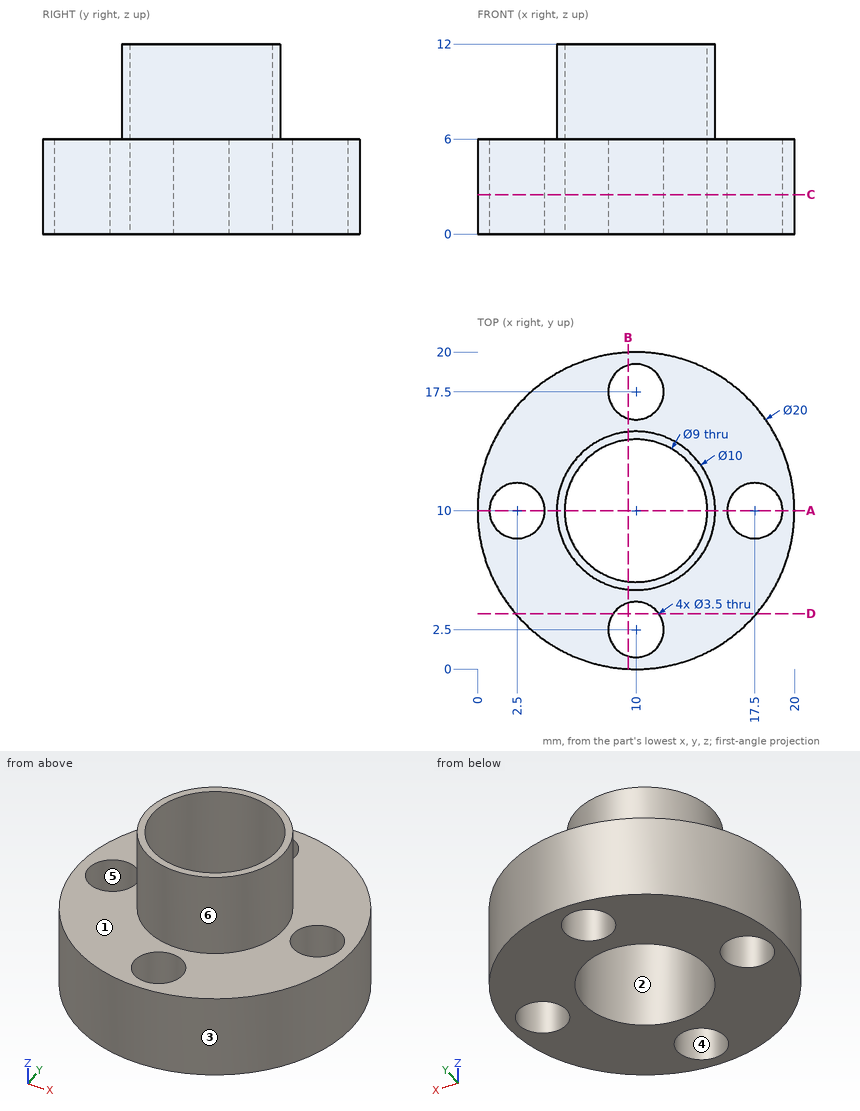
Answer from the drawing. Dimensions are ordinates in mm from the lowest x, y and z of the part. A direction names the side the tool comes from. Coordinates: 2 decimals unless noted, no trailing zeros. Loops run counter-clockwise (first coordinate to the right, second up) from the corner with the lowest first, then second, coordinate; pieces in that order, holes last. Notation, with made-up numbers: (-21, 4.25) -> (-11, 4.25) arc R20 ccw to (-11, 20.25) -> close; hole circle Ø2 at (-5, 75). An arc over 180 degrees is marked (long way). Answer in a Markdown table with one row per item.
Item 1: Straight lines are drawn through the part: line 1 along Y through (x, z) = (10, 3.6); line 2 along Y through (x, z) = (11, 4); line 3 along Z through (x, y) = (13.75, 15). For each, find the intervals that lie inside material, in ascending order. Write a range as [from, to].
Returned:
| item | result |
|---|---|
| line 1 | y = [0, 0.75], [4.25, 5.5], [14.5, 15.75], [19.25, 20] |
| line 2 | y = [0.05, 1.06], [3.94, 5.61], [14.39, 16.06], [18.94, 19.95] |
| line 3 | z = [0, 6] |
Item 2: A cutting plane is placed at D-D on y = 3.5. Determine the outline of the cut face in (x, z).
Returned:
| item | result |
|---|---|
| outline | (2.4, 0) -> (8.56, 0) -> (8.56, 6) -> (2.4, 6) -> close; (11.44, 0) -> (17.6, 0) -> (17.6, 6) -> (11.44, 6) -> close |
Item 3: Each of these flat-tipped pins is pushed along its axis until it touches: P1, Ø5, axis at x = 11, y = 2, coming from the +Z side; P2, Ø3, axis at y = 14.5, z = 3.5, coming from the +X side; P3, Ø1.5, axis at x = 5.5, z = 8.5, coming from the +Y side. Where does it stop, or does it pass through?
Returned:
| item | result |
|---|---|
| P1 | stops at z = 6 |
| P2 | stops at x = 19.54 |
| P3 | stops at y = 13.31 |
Item 4: For a pull along Y with two mould halves and no side action, classify the marked faces 1, 2, 3 and 4 as released by +Y, released by -Y, zero draft, split by the parting line, or undercut.
Returned:
| item | result |
|---|---|
| face 1 | zero draft |
| face 2 | undercut |
| face 3 | split by the parting line |
| face 4 | undercut |
Item 5: A cutting plane is placed at A-A on y = 10. Determine the outline of the cut face in (x, z), plus the area to 3 significant figures.
Returned:
| item | result |
|---|---|
| outline | (0, 0) -> (0.75, 0) -> (0.75, 6) -> (0, 6) -> close; (4.25, 0) -> (5.5, 0) -> (5.5, 12) -> (5, 12) -> (5, 6) -> (4.25, 6) -> close; (14.5, 0) -> (15.75, 0) -> (15.75, 6) -> (15, 6) -> (15, 12) -> (14.5, 12) -> close; (19.25, 0) -> (20, 0) -> (20, 6) -> (19.25, 6) -> close |
| area | 30.0 mm^2 |
Item 6: A cutting plane is placed at C-C on z = 2.5. Determine the outline of the cut face in (x, y), plus the area to 3 significant figures.
Returned:
| item | result |
|---|---|
| outline | circle Ø20 at (10, 10); hole circle Ø3.5 at (2.5, 10); hole circle Ø9 at (10, 10); hole circle Ø3.5 at (10, 2.5); hole circle Ø3.5 at (10, 17.5); hole circle Ø3.5 at (17.5, 10) |
| area | 212 mm^2 |
Item 7: A cutting plane is placed at B-B on x = 9.5. Determine the outline of the cut face in (y, z).
Returned:
| item | result |
|---|---|
| outline | (0.01, 0) -> (0.82, 0) -> (0.82, 6) -> (0.01, 6) -> close; (4.18, 0) -> (5.53, 0) -> (5.53, 12) -> (5.03, 12) -> (5.03, 6) -> (4.18, 6) -> close; (14.47, 0) -> (15.82, 0) -> (15.82, 6) -> (14.97, 6) -> (14.97, 12) -> (14.47, 12) -> close; (19.18, 0) -> (19.99, 0) -> (19.99, 6) -> (19.18, 6) -> close |
Item 8: For the marked faces 5 and 6, determine the directions among +Z, -Z, +X, -X, +Y, -Y from which every point of the face is accessible in a straight line to the end or side of a thin tool.
Returned:
| item | result |
|---|---|
| face 5 | +Z, -Z |
| face 6 | +Z |
